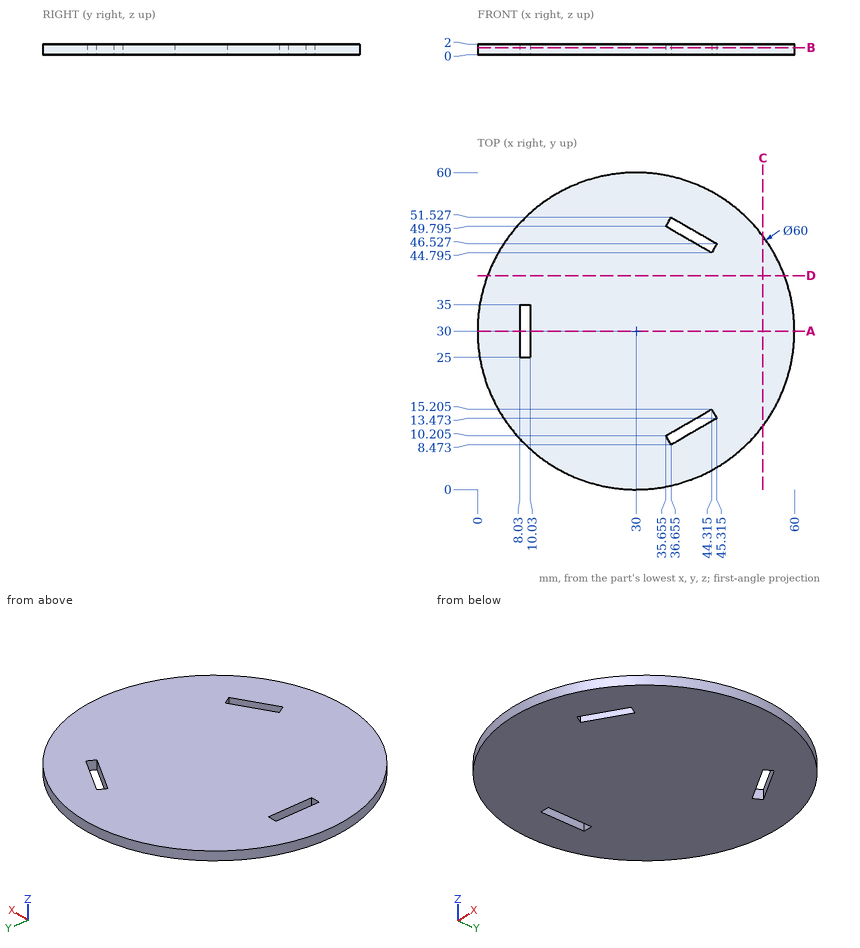
Print and shaded views of the part. All mm, measured from the part's lowest x, y and z. Coordinates: 2 decimals unless noted, no trailing zeros. Loops run counter-clockwise (first coordinate to the right, second up) from the corner with the lowest first, then second, coordinate; pieces in that order, holes last. Notation, with made-up numbers: (65, 15.25) -> (123, 15.25) arc R24 cw to (123, 50.25) -> close; hole circle Ø10 at (54.25, -36.5). An arc over 180 degrees is marked (long way). Use a Markdown table: item, result. Add a question column.
Item 1: Flat gauge pins, fed straight in: P1, Ø1, axis at x = 24.5, z = 1, coming from the +Y side; P2, Ø1, axis at y = 28, z = 0.5, coming from the +X side; P3, Ø0.6, axis at x = 9, z = 1, coming from the -Y side (1 decimal). Where does each tip first touch, or does it go through?
Item 2: Band-saw the part on B-B on z = 1.3. Write the cut outline in (x, y) (1 decimal).
Item 3: Band-saw the part on A-A on y = 30. Write the cut outline in (x, z), plus the area to 3 significant figures.
Item 4: Probe probe 1 along X at (y, z) = (32.5, 0.4) (1 decimal); probe 2 along X at (y, z) = (29, 0.3); probe 3 along X at (y, z) = (22.5, 0.85). List the from-to ranges inside material, lowest first.
Item 5: Band-saw the part on D-D on y = 40.5. Write the cut outline in (x, z).
Item 6: Band-saw the part on C-C on x = 54. Write the cut outline in (y, z).
Geometry says:
| question | item | result |
|---|---|---|
| 1 | P1 | y = 59.58 |
| 1 | P2 | x = 59.96 |
| 1 | P3 | y = 8.3 |
| 2 | outline | circle Ø60 at (30, 30); hole (8, 25) -> (10, 25) -> (10, 35) -> (8, 35) -> close; hole (35.7, 10.2) -> (36.7, 8.5) -> (45.3, 13.5) -> (44.3, 15.2) -> close; hole (35.7, 49.8) -> (44.3, 44.8) -> (45.3, 46.5) -> (36.7, 51.5) -> close |
| 3 | outline | (0, 0) -> (8.03, 0) -> (8.03, 2) -> (0, 2) -> close; (10.03, 0) -> (60, 0) -> (60, 2) -> (10.03, 2) -> close |
| 3 | area | 116 mm² |
| 4 | probe 1 | 0.1 to 8, 10 to 59.9 |
| 4 | probe 2 | 0.02 to 8.03, 10.03 to 59.98 |
| 4 | probe 3 | 0.95 to 59.05 |
| 5 | outline | (1.9, 0) -> (58.1, 0) -> (58.1, 2) -> (1.9, 2) -> close |
| 6 | outline | (12, 0) -> (48, 0) -> (48, 2) -> (12, 2) -> close |
